Autodesk Inventor part; units mm, degrees
ref_plane "YZ Plane" through (0, 0, 0) normal (1, 0, 0) x (0, 1, 0)
ref_plane "XZ Plane" through (0, 0, 0) normal (0, 1, 0) x (-1, 0, 0)
ref_plane "XY Plane" through (0, 0, 0) normal (0, 0, 1) x (1, 0, 0)
sketch "スケッチ1" plane through (0, 0, 0) normal (0, 0, 1) x (1, 0, 0)
  line L0 (-10, 5) -> (10, 5)
  line L1 (10, 5) -> (10, -5)
  line L2 (10, -5) -> (-10, -5)
  line L3 (-10, -5) -> (-10, 5)
  line L4 (-10, 5) -> (10, -5) construction
  line L5 (10, 5) -> (-10, -5) construction
  point P0 (0, 0)
  dimension "d0" = 20
  dimension "d1" = 10
extrude "押し出し1" add sketch "スケッチ1" along normal mid plane 55
sketch "スケッチ2" plane through (0, 0, 27.5) normal (0, 0, 1) x (1, 0, 0)
  line L0 (-10, -5) -> (10, -5)
  line L1 (-10, 5) -> (-10, -5)
  line L2 (10, -5) -> (10, 5)
  point P0 (0, 0)
  point P1 (-5, 0)
  point P2 (5, 0)
  dimension "d4" = 5
  dimension "d5" = 5
  dimension "d6" = 5
  dimension "d7" = 5
hole "穴1" at (-5, 0, 27.5) at (5, 0, 27.5) direction (0, 0, -1) diameter 2.459 depth 8.8 tip angle 118
sketch "スケッチ3" plane through (0, 0, -27.5) normal (0, 0, -1) x (-1, 0, 0)
  line L0 (-10, -5) -> (10, -5)
  line L1 (10, -5) -> (10, 5)
  line L2 (10, 5) -> (-10, 5)
  line L3 (-10, 5) -> (-10, -5)
  circle A0 centre (-5, 0) radius 1.2295
  circle A1 centre (5, 0) radius 1.2295
  point P0 (0, 0)
hole "穴2" at (5, 0, -27.5) at (-5, 0, -27.5) direction (0, 0, 1) diameter 2.459 depth 8.8 tip angle 118
sketch "スケッチ5" plane through (-10, 5, 27.5) normal (0, 1, 0) x (1, 0, 0)
  line L0 (20, 55) -> (20, 0)
  line L1 (0, 55) -> (20, 55)
  point P0 (10, 27.5)
  point P1 (15, 27.5)
  point P2 (5, 27.5)
  dimension "d22" = 5
  dimension "d23" = 10
  dimension "d24" = 27.5
  dimension "d25" = 27.5
hole "穴3" at (5, 5, 0) at (-5, 5, 0) direction (0, -1, 0) diameter 5.5 end through all
fillet "フィレット1" radius 1 4 edges at (-10, 5, 0) (10, 5, 0) (10, -5, 0) (-10, -5, 0)
properties part number "center_part"
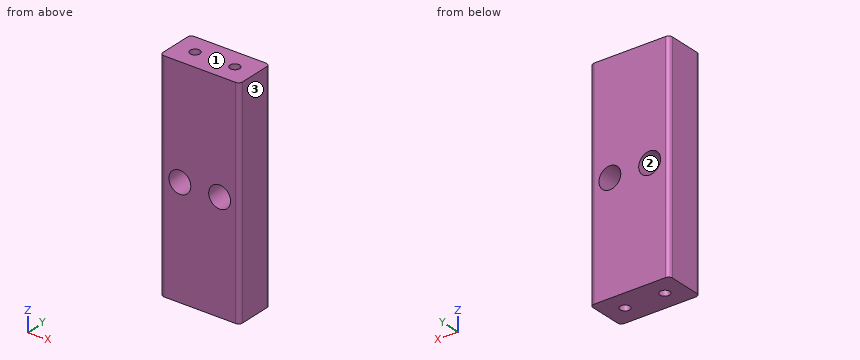
For this review, take the finished solid that the model builds, in its own axes (mm). Face numbers are marked on the shaded views. Give positions to 0.01 mm unless a question says otherwise; leave off trailing zeros. Loops run counter-clockwise (first coordinate to the right, second up) from the corner with the lowest first, then second, coordinate; pieces in that order, holes last.
Item 1: For line 1 along X through (y, z) = (0, 22.5); line 2 along Z through (x, y) = (-5, -1.75); line 3 along Y through (x, z) = (5, -21.25), list the stretches that pass through material, from the lowest coordinate up.
Item 2: Take a section at D-D, the plane y = 2.5. State the section outline as (x, z) points.
Item 3: Draft analysis for pull direction X (two halves, no side actions). For the marked faces 1, 2 and 3, state which applies: +X half, -X half, draft (parallel to the pull), parting line (faces both ways), or undercut.
Item 4: Take a section at A-A, the plane z = 0. State the section outline as (x, y) points, and give its area (3 significant figures).
Item 5: Take a section at C-C, the plane z = -21.5. State the section outline as (x, y) points.
Item 6: Insertion check: pin 1 (2 mm diameter, centred on x = 5, y = 0, fed in from +Z); pin 2 (4.5 mm diameter, centred on x = 5, z = 0, fed in from +Y); pin 3 (1.5 mm diameter, centred on x = -5, y = 0, fed in from -Z). Each pin has a flat end and moves straight along its axis. Give the tip position at first contact, or say it passes through.
Item 7: Take a section at B-B, the plane x = -3.25. State the section outline as (y, z) points.
Calculated:
1. line 1: x = -10 to -6.23, -3.77 to 3.77, 6.23 to 10
1. line 2: z = -27.5 to -2.75, 2.75 to 27.5
1. line 3: y = -5 to -1.23, 1.23 to 5
2. outline: (-10, -27.5) - (10, -27.5) - (10, 27.5) - (-10, 27.5) - close; hole circle Ø5.5 at (-5, 0); hole circle Ø5.5 at (5, 0)
3. face 1: draft
3. face 2: undercut
3. face 3: +X half
4. outline: (-10, -4) arc R1 ccw to (-9, -5) - (-7.75, -5) - (-7.75, 5) - (-9, 5) arc R1 ccw to (-10, 4) - close; (-2.25, -5) - (2.25, -5) - (2.25, 5) - (-2.25, 5) - close; (7.75, -5) - (9, -5) arc R1 ccw to (10, -4) - (10, 4) arc R1 ccw to (9, 5) - (7.75, 5) - close
4. area: 89.1 mm2
5. outline: (-10, -4) arc R1 ccw to (-9, -5) - (9, -5) arc R1 ccw to (10, -4) - (10, 4) arc R1 ccw to (9, 5) - (-9, 5) arc R1 ccw to (-10, 4) - close; hole circle Ø2.46 at (-5, 0); hole circle Ø2.46 at (5, 0)
6. pin 1: stops at z = 18.56
6. pin 2: passes through
6. pin 3: stops at z = -18.41
7. outline: (-5, -27.5) - (5, -27.5) - (5, -2.12) - (-5, -2.12) - close; (-5, 2.12) - (5, 2.12) - (5, 27.5) - (-5, 27.5) - close
